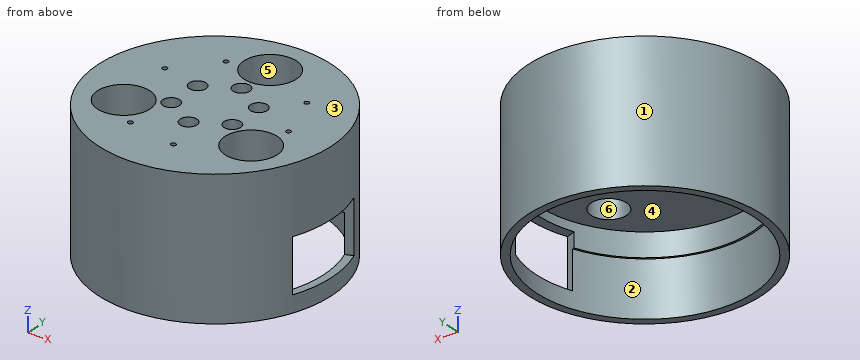
from build123d import *

# Parameters (mm, degrees)
SKETCH_1_R               = 59
F_01_BODY_D118_DEPTH     = 69.5
SKETCH_2_R               = 55
F_02_BORE_D110_DEPTH     = 28
SKETCH_3_R               = 54
F_03_BORE_D108_DEPTH     = 12
SKETCH_4_R               = 4.25
F_04_HOLES_6_D8_5_DEPTH  = 24
SKETCH_5_R               = 13.25
F_05_LOBES_3_D26_5_DEPTH = 19.5
SKETCH_6_R               = 9
F_06_THRU_3_D18_DEPTH    = 10
F_07_WINDOW_27X40_DEPTH  = 27
SKETCH_8_R               = 1.25
F_08_TAP_9_M3_DEPTH      = 6


with BuildPart() as part:
    # 草图1 → 01_BODY_D118 (new body)
    with BuildSketch(Plane.XY):
        Circle(SKETCH_1_R)
    extrude(amount=F_01_BODY_D118_DEPTH)

    # 草图2 → 02_BORE_D110 (cut)
    with BuildSketch(Plane.XY):
        Circle(SKETCH_2_R)
    extrude(amount=F_02_BORE_D110_DEPTH, mode=Mode.SUBTRACT)

    # 草图3 → 03_BORE_D108 (cut)
    with BuildSketch(Plane.XY.offset(28)):
        Circle(SKETCH_3_R)
    extrude(amount=F_03_BORE_D108_DEPTH, mode=Mode.SUBTRACT)

    # 草图4 → 04_HOLES_6_D8.5 (cut)
    with BuildSketch(Plane.XY.offset(69.5)):
        with Locations((15.588457268, 9)):
            Circle(SKETCH_4_R)
        with Locations((0, 18)):
            Circle(SKETCH_4_R)
        with Locations((-15.588457268, 9)):
            Circle(SKETCH_4_R)
        with Locations((-15.588457268, -9)):
            Circle(SKETCH_4_R)
        with Locations((0, -18)):
            Circle(SKETCH_4_R)
        with Locations((15.588457268, -9)):
            Circle(SKETCH_4_R)
    extrude(amount=-F_04_HOLES_6_D8_5_DEPTH, mode=Mode.SUBTRACT)

    # 草图5 → 05_LOBES_3_D26.5 (cut)
    with BuildSketch(Plane.XY.offset(69.5)):
        with Locations((0, 37.5)):
            Circle(SKETCH_5_R)
        with Locations((-32.475952642, -18.75)):
            Circle(SKETCH_5_R)
        with Locations((32.475952642, -18.75)):
            Circle(SKETCH_5_R)
    extrude(amount=-F_05_LOBES_3_D26_5_DEPTH, mode=Mode.SUBTRACT)

    # 草图6 → 06_THRU_3_D18 (cut)
    with BuildSketch(Plane.XY.offset(50)):
        with Locations((0, 37.5)):
            Circle(SKETCH_6_R)
        with Locations((-32.475952642, -18.75)):
            Circle(SKETCH_6_R)
        with Locations((32.475952642, -18.75)):
            Circle(SKETCH_6_R)
    extrude(amount=-F_06_THRU_3_D18_DEPTH, mode=Mode.SUBTRACT)

    # 草图7 → 07_WINDOW_27X40 (cut)
    with BuildSketch(Plane.XY.offset(8.5)):
        with BuildLine():
            Line((55.179875165, 20.884955752), (50.503614558, 19.115044248))
            ThreePointArc((50.503614558, 19.115044248), (54, 0), (50.503614558, -19.115044248))
            Line((50.503614558, -19.115044248), (55.179875165, -20.884955752))
            ThreePointArc((55.179875165, -20.884955752), (59, 0), (55.179875165, 20.884955752))
        make_face()
    extrude(amount=F_07_WINDOW_27X40_DEPTH, mode=Mode.SUBTRACT)

    # 草图8 → 08_TAP_9_M3 (cut)
    with BuildSketch(Plane.XY.offset(69.5)):
        with Locations((-18.75, 32.475952642)):
            Circle(SKETCH_8_R)
        with Locations((-35.238473279, 12.825755375)):
            Circle(SKETCH_8_R)
        with Locations((-35.238473279, -12.825755375)):
            Circle(SKETCH_8_R)
        with Locations((-18.75, -32.475952642)):
            Circle(SKETCH_8_R)
        with Locations((6.511806663, -36.930290738)):
            Circle(SKETCH_8_R)
        with Locations((28.726666617, -24.104535363)):
            Circle(SKETCH_8_R)
        with Locations((37.5, 0)):
            Circle(SKETCH_8_R)
        with Locations((28.726666617, 24.104535363)):
            Circle(SKETCH_8_R)
        with Locations((6.511806663, 36.930290738)):
            Circle(SKETCH_8_R)
    extrude(amount=-F_08_TAP_9_M3_DEPTH, mode=Mode.SUBTRACT)


solid = part.part
Input: part model. Units: mm. Frame: model coordinates. Face numbers are marked on the shaded views. A direction names the side the tool comes from. Give positions to 0.01 mm unless a question says otherwise; leave off trailing zeros. Write each loop counter-clockwise with the first axis right and the second up, starting at its lowest first coordinate (ties: lowest second). Pieces come first, ordered by that corner, then holes.
Q1. Section C-C, the plane z = 32.5. Output: boundary loops of the cut face in (x, y).
Q2. Set-up query: the marked faces 4, 5 and 6. Return all of +Z, -Z, +X, -X, +Y, -Y with unobstructed straight access to the full face (end or side cutting, diameter ignored); none if empty.
Q3. Section D-D, the plane y = 9. Output: boundary loops of the cut face in (x, z).
Q4. Pull-direction query (X, two-part tool) for the marked faces 1, 2 and 3; classes: pulls with the +X half, pulls with the -X half, needs draft (parallel to the pull), parting line crosses it, or undercut.
Q5. Section A-A, the plane y = 37.5. Output: boundary loops of the cut face in (x, z), plus the area to 3 significant figures.
Q6. Material intervals for probe 1 along Y at (x, z) = (0, 62.5); probe 2 along X at (y, z) = (12, 52); probe 3 along Z at (x, y) = (16.5, 43.5), sorted ascending.
Q7. Section B-B, the plane z = 53. State how many separate pieces and enclosed holes the cut face has, plus the area to 3 significant figures.
Q8. First-contact query: P1, Ø1.5, axis at y = -46, z = 41.5, coming from the +X side; P2, Ø0.8, axis at x = 6, y = -37, coming from the +Z side; P3, Ø2.5, axis at x = -15.5, y = -7.5, coming from the +Z side. Flat tips, straight axial feed; report the tip coordinate or a pass-through.
Filled in:
1. outline: (50.5, -19.12) arc R54 cw (long way) to (50.5, 19.12) - (55.18, 20.88) arc R59 ccw (long way) to (55.18, -20.88) - close
2. face 4: -Z
2. face 5: +Z
2. face 6: +Z, -Z
3. outline: (-58.31, 0) - (-54.26, 0) - (-54.26, 28) - (-53.24, 28) - (-53.24, 40) - (53.24, 40) - (53.24, 35.5) - (58.31, 35.5) - (58.31, 69.5) - (19.84, 69.5) - (19.84, 45.5) - (11.34, 45.5) - (11.34, 69.5) - (-11.34, 69.5) - (-11.34, 45.5) - (-19.84, 45.5) - (-19.84, 69.5) - (-58.31, 69.5) - close; (54.26, 0) - (58.31, 0) - (58.31, 8.5) - (54.26, 8.5) - close
4. face 1: parting line crosses it
4. face 2: undercut
4. face 3: needs draft
5. outline: (-45.55, 0) - (-40.23, 0) - (-40.23, 28) - (-38.86, 28) - (-38.86, 40) - (-9, 40) - (-9, 50) - (-13.25, 50) - (-13.25, 69.5) - (-45.55, 69.5) - close; (9, 40) - (38.86, 40) - (38.86, 28) - (40.23, 28) - (40.23, 0) - (45.55, 0) - (45.55, 69.5) - (13.25, 69.5) - (13.25, 50) - (9, 50) - close
5. area: 2,450 mm2
6. probe 1: y = -59 to -22.25, -13.75 to 13.75, 22.25 to 24.25, 50.75 to 59
6. probe 2: x = -57.77 to -18.6, -12.58 to 12.58, 18.6 to 57.77
6. probe 3: z = 40 to 69.5
7. separate pieces: 1
7. enclosed holes: 9
7. area: 8,940 mm2
8. P1: stops at x = 37.86
8. P2: stops at z = 63.5
8. P3: stops at z = 45.5
